Read the model definition and answer for the solid it produces. Units are mm, in the model's axes. Face numbers are marked on the shaded views. A direction names the side the tool comes from. Give positions to 0.01 mm unless a question says otherwise; leave off trailing zeros. Write each loop counter-clockwise with the first axis right and the second up, starting at its lowest first coordinate (ties: lowest second). Pieces come first, ordered by that corner, then holes. Notation, with made-up numbers: M -36,-31 L -7,-31 A25 ccw -7,-13 Z; hole C 42.5,68.25 d4. An arc over 180 degrees is marked long. Use a Markdown table: item, result. Add a question column.
Item 1: A cutting plane is placed at A-A on z = 6.25. Determine the outline of the cut face in (x, y).
Item 2: The mould has two halves that part along X. Classify the marked faces 1, 2, 3 and 4: pulls with the +X half, pulls with the -X half, needs draft (parallel to the pull), parting line crosses it, or undercut.
Item 3: For the marked faces 5, 6 and 7, determine the directions among +Z, -Z, +X, -X, +Y, -Y from which every point of the face is accessible in a straight line to the end or side of a thin tool.
Item 4: Consider probe 1 along Y at (x, z) = (0, 4.5); probe 2 along Y at (x, z) = (3, 4.25); probe 3 along X at (y, z) = (-37, 0.5). Determine where each line is inside the solid, lowest interval first. Write a range as [from, to].
Item 5: A cutting plane is placed at D-D on y = 17.5. Determine the outline of the cut face in (x, z), then the cut area to 3 significant figures.
Item 6: A cutting plane is placed at B-B on x = 0. Determine the outline of the cut face in (y, z), then the cut area to 3 significant figures.
Item 7: A cutting plane is placed at C-C on x = 30. Determine the outline of the cut face in (y, z).
Item 8: Given P1, Ø12, axis at x = 0, y = 36.4, coming from the -Z side; P2, Ø4, axis at x = -27.5, z = 3.5, coming from the +Y side; P3, Ø2, axis at x = 30, z = 5, coming from the -Y side; P4, Ø4, axis at y = 29.5, z = 6.5, coming from the -X side, each flat-ended and moving along its own axis, determine where each tip first touches the part or whether it passes through.
from build123d import *

# Parameters (mm, degrees)
F0_R     = 9.811337
F1_DEPTH = 7.5
F2_R     = 5.08
F3_R     = 5.08
F4_R     = 5.08
F5_R     = 5.08


with BuildPart() as f1:
    # F0 (on Top) → F1 (new body)
    with BuildSketch(Plane.XY):
        with BuildLine():
            ThreePointArc((-13.557643, 36.400266), (0, 22.842624), (13.557643, 36.400266))
            ThreePointArc((13.557643, 36.400266), (0, 49.957909), (-13.557643, 36.400266))
        make_face()
        with Locations((0, 36.400266)):
            Circle(F0_R, mode=Mode.SUBTRACT)
        with BuildLine():
            Line((13.557643, 13.557643), (13.557643, 36.400266))
            ThreePointArc((13.557643, 36.400266), (0, 22.842624), (-13.557643, 36.400266))
            Line((-13.557643, 36.400266), (-13.557643, 13.557643))
            Line((-13.557643, 13.557643), (-36.400266, 13.557643))
            ThreePointArc((-36.400266, 13.557643), (-26.813565, 9.586701), (-22.842624, 0))
            ThreePointArc((-22.842624, 0), (-26.813565, -9.586701), (-36.400266, -13.557643))
            Line((-36.400266, -13.557643), (-13.557643, -13.557643))
            Line((-13.557643, -13.557643), (-13.557643, -36.400266))
            ThreePointArc((-13.557643, -36.400266), (0, -22.842624), (13.557643, -36.400266))
            Line((13.557643, -36.400266), (13.557643, -13.557643))
            Line((13.557643, -13.557643), (36.400266, -13.557643))
            ThreePointArc((36.400266, -13.557643), (22.842624, 0), (36.400266, 13.557643))
            Line((36.400266, 13.557643), (13.557643, 13.557643))
        make_face()
        Circle(F0_R, mode=Mode.SUBTRACT)
        with BuildLine():
            ThreePointArc((49.957909, 0), (45.986968, 9.586701), (36.400266, 13.557643))
            ThreePointArc((36.400266, 13.557643), (22.842624, 0), (36.400266, -13.557643))
            ThreePointArc((36.400266, -13.557643), (45.986968, -9.586701), (49.957909, 0))
        make_face()
        with Locations((36.400266, 0)):
            Circle(F0_R, mode=Mode.SUBTRACT)
        with BuildLine():
            ThreePointArc((-22.842624, 0), (-26.813565, 9.586701), (-36.400266, 13.557643))
            ThreePointArc((-36.400266, 13.557643), (-49.957909, 0), (-36.400266, -13.557643))
            ThreePointArc((-36.400266, -13.557643), (-26.813565, -9.586701), (-22.842624, 0))
        make_face()
        with Locations((-36.400266, 0)):
            Circle(F0_R, mode=Mode.SUBTRACT)
        with BuildLine():
            ThreePointArc((-13.557643, -36.400266), (0, -49.957909), (13.557643, -36.400266))
            ThreePointArc((13.557643, -36.400266), (0, -22.842624), (-13.557643, -36.400266))
        make_face()
        with Locations((0, -36.400266)):
            Circle(F0_R, mode=Mode.SUBTRACT)
    extrude(amount=F1_DEPTH)

    # F2
    f2_edges = [f1.edges().sort_by_distance(p)[0] for p in [
        (-13.557643, 13.557643, 3.75),
    ]]
    fillet(f2_edges, radius=F2_R)

    # F3
    f3_edges = [f1.edges().sort_by_distance(p)[0] for p in [
        (13.557643, 13.557643, 3.75),
    ]]
    fillet(f3_edges, radius=F3_R)

    # F4
    f4_edges = [f1.edges().sort_by_distance(p)[0] for p in [
        (-13.557643, -13.557643, 3.75),
    ]]
    fillet(f4_edges, radius=F4_R)

    # F5
    f5_edges = [f1.edges().sort_by_distance(p)[0] for p in [
        (13.557643, -13.557643, 3.75),
    ]]
    fillet(f5_edges, radius=F5_R)


solid = f1.part
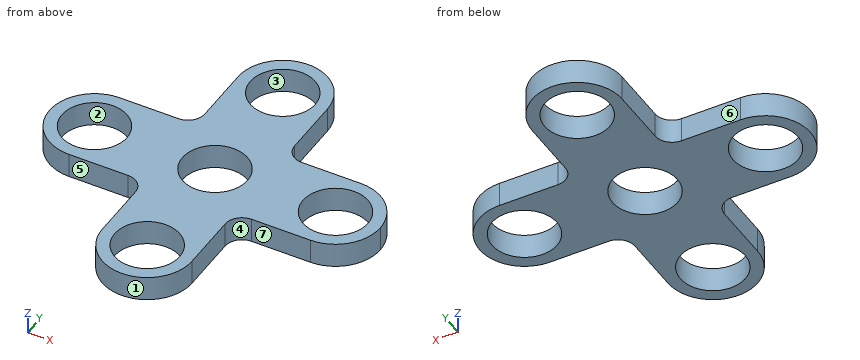
Filled in:
| question | item | result |
|---|---|---|
| 1 | outline | M -36.4,-13.56 L -18.64,-13.56 A5.08 cw -13.56,-18.64 L -13.56,-36.4 A13.56 ccw 13.56,-36.4 L 13.56,-18.64 A5.08 cw 18.64,-13.56 L 36.4,-13.56 A13.56 ccw 49.96,0 A13.56 ccw 36.4,13.56 L 18.64,13.56 A5.08 cw 13.56,18.64 L 13.56,36.4 A13.56 ccw -13.56,36.4 L -13.56,18.64 A5.08 cw -18.64,13.56 L -36.4,13.56 A13.56 ccw Z; hole C -36.4,0 d19.62; hole C 0,-36.4 d19.62; hole C 0,0 d19.62; hole C 0,36.4 d19.62; hole C 36.4,0 d19.62 |
| 2 | face 1 | parting line crosses it |
| 2 | face 2 | undercut |
| 2 | face 3 | undercut |
| 2 | face 4 | pulls with the +X half |
| 3 | face 5 | +Z, -Z, -X, -Y |
| 3 | face 6 | +Z, -Z, -X, +Y |
| 3 | face 7 | +Z, -Z, +X, -Y |
| 4 | probe 1 | [-49.96, -46.21], [-26.59, -9.81], [9.81, 26.59], [46.21, 49.96] |
| 4 | probe 2 | [-49.62, -45.74], [-27.06, -9.34], [9.34, 27.06], [45.74, 49.62] |
| 4 | probe 3 | [-13.54, -9.79], [9.79, 13.54] |
| 5 | outline | M -13.69,0 L 13.69,0 L 13.69,7.5 L -13.69,7.5 Z |
| 5 | area | 205 mm² |
| 6 | outline | M -49.96,0 L -46.21,0 L -46.21,7.5 L -49.96,7.5 Z; M -26.59,0 L -9.81,0 L -9.81,7.5 L -26.59,7.5 Z; M 9.81,0 L 26.59,0 L 26.59,7.5 L 9.81,7.5 Z; M 46.21,0 L 49.96,0 L 49.96,7.5 L 46.21,7.5 Z |
| 6 | area | 308 mm² |
| 7 | outline | M -13.56,0 L -7.44,0 L -7.44,7.5 L -13.56,7.5 Z; M 7.44,0 L 13.56,0 L 13.56,7.5 L 7.44,7.5 Z |
| 8 | P1 | through |
| 8 | P2 | y = 13.56 |
| 8 | P3 | y = -13.56 |
| 8 | P4 | x = -13.56 |
